Drawing for the job (mm, zero at the part's lowest x, y, z). Give positions to 0.01 mm unless a question says otherwise; leave off trailing zeros. Loops run counter-clockwise (first coordinate to the right, second up) from the corner with the lowest first, then second, coordinate; pieces in that order, holes last. Notation, with made-up numbers: (-39, 7.5) -> (15, 7.5) arc R28 ccw to (15, 37.5) -> close; hole circle Ø7 at (55, 33). An arc over 180 degrees is marked (long way). Answer in a Markdown table with one row per item. Add a question column.
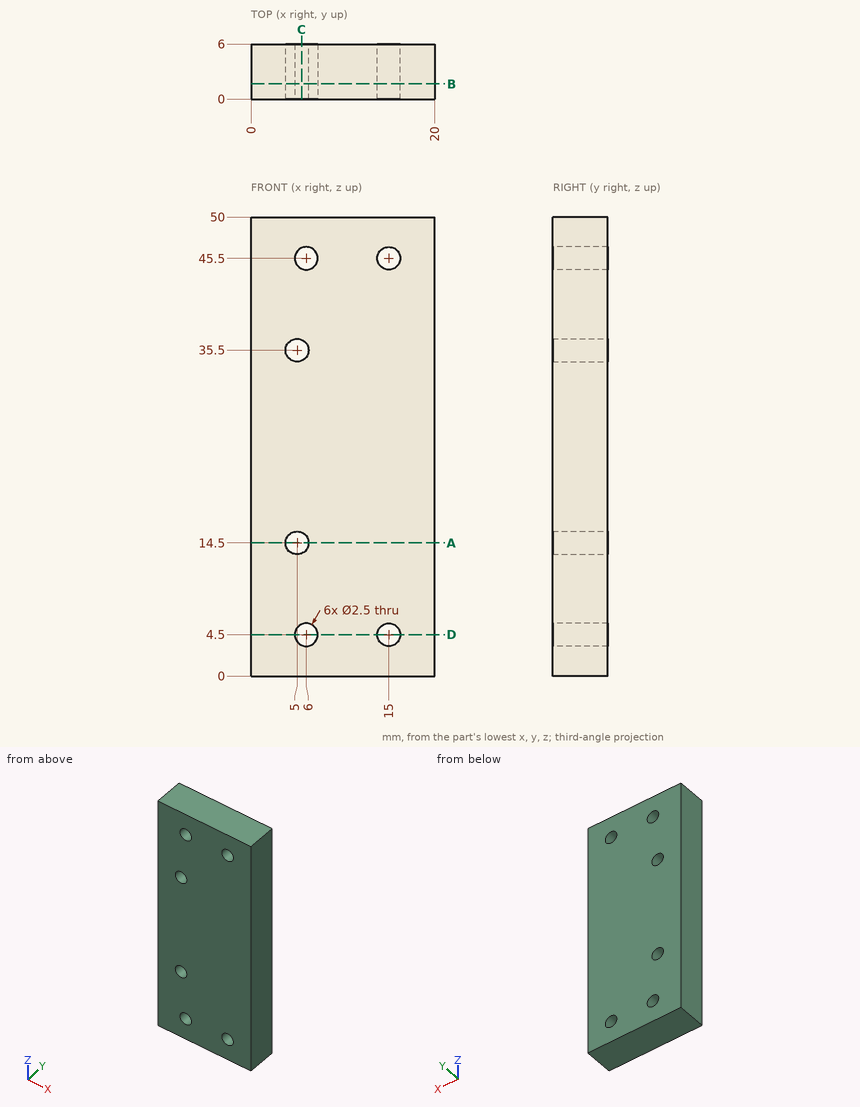
(1) Saw through at C-C, the plane x = 5.5. List the corners of the cut face in (y, z), then the cut area to 3 significant figures.
(2) Wall check: line 1 along Z through (x, y) = (15, 1.7); line 2 along X through (y, z) = (4.3, 3.5); line 3 along Z through (x, y) = (14.25, 5.35). Give the ranges that are in metal, low to high. Write a range as from..to.
(3) Saw through at D-D, the plane z = 4.5. List the corners of the cut face in (x, y).
(4) Saw through at A-A, the plane z = 14.5. List the corners of the cut face in (x, y).
(5) Saw through at B-B, the plane y = 1.65. List the corners of the cut face in (x, z), then the cut area to 3 significant figures.
Worked answers:
| question | item | result |
|---|---|---|
| 1 | outline | (0, 0) -> (6, 0) -> (6, 3.35) -> (0, 3.35) -> close; (0, 5.65) -> (6, 5.65) -> (6, 13.35) -> (0, 13.35) -> close; (0, 15.65) -> (6, 15.65) -> (6, 34.35) -> (0, 34.35) -> close; (0, 36.65) -> (6, 36.65) -> (6, 44.35) -> (0, 44.35) -> close; (0, 46.65) -> (6, 46.65) -> (6, 50) -> (0, 50) -> close |
| 1 | area | 245 mm^2 |
| 2 | line 1 | 0..3.25, 5.75..44.25, 46.75..50 |
| 2 | line 2 | 0..5.25, 6.75..14.25, 15.75..20 |
| 2 | line 3 | 0..3.5, 5.5..44.5, 46.5..50 |
| 3 | outline | (0, 0) -> (4.75, 0) -> (4.75, 6) -> (0, 6) -> close; (7.25, 0) -> (13.75, 0) -> (13.75, 6) -> (7.25, 6) -> close; (16.25, 0) -> (20, 0) -> (20, 6) -> (16.25, 6) -> close |
| 4 | outline | (0, 0) -> (3.75, 0) -> (3.75, 6) -> (0, 6) -> close; (6.25, 0) -> (20, 0) -> (20, 6) -> (6.25, 6) -> close |
| 5 | outline | (0, 0) -> (20, 0) -> (20, 50) -> (0, 50) -> close; hole circle Ø2.5 at (5, 14.5); hole circle Ø2.5 at (5, 35.5); hole circle Ø2.5 at (6, 4.5); hole circle Ø2.5 at (6, 45.5); hole circle Ø2.5 at (15, 4.5); hole circle Ø2.5 at (15, 45.5) |
| 5 | area | 971 mm^2 |
